```python
from build123d import *

# Parameters (mm, degrees)
SKETCH_1_R           = 22.5
SKETCH_1_R_2         = 17.5
EXTRUDE_1_DEPTH      = 15
EXTRUDE_2_REACH      = 166.735
EXTRUDE_2_END_RADIUS = 22.5
SKETCH_2_R           = 5
SKETCH_3_W           = 25
SKETCH_3_H           = 25
EXTRUDE_3_DEPTH      = 5


with BuildPart() as part:
    # 草图1 → 凸台-拉伸1 (new body)
    with BuildSketch(Plane.XY):
        Circle(SKETCH_1_R)
        Circle(SKETCH_1_R_2, mode=Mode.SUBTRACT)
    extrude(amount=EXTRUDE_1_DEPTH)

    # 凸台-拉伸2: up to this cylinder (the profile starts outside it)
    extrude_2_end = Plane(origin=(0, 0, 7.5), z_dir=(0, 0, -1)) * Cylinder(EXTRUDE_2_END_RADIUS, 379.47, mode=Mode.PRIVATE)
    # 草图2 → 凸台-拉伸2 (add, up to the surface)
    with BuildSketch(Plane(origin=(0, -140, 0), x_dir=(1, 0, 0), z_dir=(0, 1, 0)), mode=Mode.PRIVATE) as extrude_2_sk1:
        with Locations(Location((0, -7.5, 0), (0, 0, 90))):
            Circle(SKETCH_2_R)
    extrude_2_tool1 = extrude(extrude_2_sk1.sketch, amount=EXTRUDE_2_REACH, mode=Mode.PRIVATE) - extrude_2_end
    add(extrude_2_tool1.solids().sort_by_distance((0, -140, 7.5))[0])

    # 草图3 → 凸台-拉伸3 (add)
    with BuildSketch(Plane.XZ.offset(140)):
        with Locations((0, 7.5)):
            Rectangle(SKETCH_3_W, SKETCH_3_H)
    extrude(amount=EXTRUDE_3_DEPTH)


solid = part.part
```
For this review, take the finished solid that the model builds, in its own axes (mm). A direction names the side the tool comes from. Give positions to 0.01 mm unless a question says otherwise; leave off trailing zeros. Write each loop counter-clockwise with the first axis right and the second up, starting at its lowest first coordinate (ties: lowest second). Pieces come first, ordered by that corner, then holes. Notation, with made-up numbers: M 69.25,54.5 L 111.25,54.5 A30 cw 111.25,78.5 Z; hole C 53.5,-6 d7. An arc over 180 degrees is marked long. Answer as a JSON object with one key per item and string values. Group by question number.
Item 1: Consider section A-A on y = 0. Write out the cut boundary in (x, z), plus the area to 3 significant figures.
Item 2: Draft analysis for pull direction Y (two halves, no side actions). For faces 1 (the flat face through (12.5, -142, 7)), 2 (the cylindrical face through (12.1, 18.97, 7.4)), 3 (the flat face through (0, -145, 8)), state which applies: +Y half, -Y half, draft (parallel to the pull), parting line (faces both ways), or undercut.
Item 3: For pin 1 Ø2.5 at (y, z) = (-143, 4.5) entering from +X; pin 2 Ø4 at (x, y) = (1, -88.5) entering from -Z; pin 3 Ø4 at (y, z) = (-30, 3.5) entering from +X, all flat-tipped, find the tip position at first contact; note any pin that passes through.
Item 4: Consider section C-C on z = 7.5. Write out the cut boundary in (x, y).
Item 5: Consider section D-D on x = 15.5. Write out the cut boundary in (y, z), plus the area to 3 significant figures.
Item 6: Tool access review of faces 4 (the cylindrical face through (-1.5, -81.8, 2.73)), 5 (the flat face through (12, -13, 0)), 6 (the flat face through (12, -13, 15)): name each direction out of +Z, -Z, +X, -X, +Y, -Y from which nothing blocks a thin tool from reaching the whole face with its end or side.
Item 7: For probe 1 along Y at (x, z) = (0, 5.25); probe 2 along Y at (x, z) = (-12, 5.25); probe 3 along Y at (x, z) = (-4, -4), list the stretches that pass through material, from the lowest coordinate up. Write a range as [from, to].
Item 8: Consider section B-B on x = 0. Write out the cut boundary in (y, z), plus the area to 3 significant figures.
Check result:
{
 "1": {"outline": "M -22.5,0 L -17.5,0 L -17.5,15 L -22.5,15 Z; M 17.5,0 L 22.5,0 L 22.5,15 L 17.5,15 Z", "area": "150 mm^2"},
 "2": {"face 1": "draft", "face 2": "undercut", "face 3": "-Y half"},
 "3": {"pin 1": "stops at x = 12.5", "pin 2": "stops at z = 2.5", "pin 3": "stops at x = 4.58"},
 "4": {"outline": "M -12.5,-145 L 12.5,-145 L 12.5,-140 L 5,-140 L 5,-21.94 A22.5 ccw long -5,-21.94 L -5,-140 L -12.5,-140 Z; hole C 0,0 d35"},
 "5": {"outline": "M -16.31,0 L -8.12,0 L -8.12,15 L -16.31,15 Z; M 8.12,0 L 16.31,0 L 16.31,15 L 8.12,15 Z", "area": "246 mm^2"},
 "6": {"face 4": "none", "face 5": "-Z, +X, -X, +Y", "face 6": "+Z, +X, -X, +Y"},
 "7": {"probe 1": "y = [-145, -17.5], [17.5, 22.5]", "probe 2": "y = [-145, -140], [-19.03, -12.74], [12.74, 19.03]", "probe 3": "y = [-145, -140]"},
 "8": {"outline": "M -145,-5 L -140,-5 L -140,2.5 L -22.5,2.5 L -22.5,0 L -17.5,0 L -17.5,15 L -22.5,15 L -22.5,12.5 L -140,12.5 L -140,20 L -145,20 Z; M 17.5,0 L 22.5,0 L 22.5,15 L 17.5,15 Z", "area": "1,450 mm^2"}
}
